Could you check a few things on this model? Use its own coordinates, in mm. A direction names the side the tool comes from. Give positions to 0.01 mm unless a question says otherwise; leave off trailing zeros. Order: outer loops, then holes, each group sorted by start corner. A loop starts at its lowest first (then second) coordinate and runs counter-clockwise, first axis right, second up. Notation, with made-up numbers: (-26, -0.5) - (32, -0.5) arc R16 cw to (32, 16.5) - close; hole circle Ø7 at (2.5, 88.5). An arc over 180 degrees is marked (long way). One line per question, with ' | ' between items. Start each with the question number.
1. I need wall thicknesses on probe 1 along Y at (x, z) = (-33.79, 13.25); probe 2 along X at (y, z) = (-1.5, 16.25) (3 decimals); probe 3 along Y at (x, z) = (-26.5, 4.75). Which ranges of each line are inside material? Lowest first, please. Write a range as from..to.
2. Imagine slicing it at C-C (z = 16). Please give me the cut outline in (x, y) (3 decimals).
3. Imagine slicing it at D-D (z = 8.75). Please give me the cut outline in (x, y) (3 decimals), and give its area (3 significant figures).
4. Which directions (+Z, -Z, +X, -X, +Y, -Y) give clear straight access to the entire face, cutting with the end or side of a thin tool? Please do faces 4 (the flat face through (-10, 10.4, 10)), 5 (the cylindrical face through (12.65, 4.19, 14.85)), 6 (the flat face through (22.395, 3, 10)).
5. Imagine slicing it at A-A (y = -4.9). Please give me the cut outline in (x, z) (3 decimals), and give its area (3 significant figures).
6. Imagine slicing it at B-B (x = 14.89). Please give me the cut outline in (y, z), and give its area (3 significant figures).
7. If we mould it in two halves opening along X, with no side actions, what happens to faces 1 (the flat face through (-41.395, 3, 10)), 2 (the flat face through (15, -5, 10)), 3 (the flat face through (-10, 11, 20))? For each: released by +X, released by -X, zero draft, split by the parting line, or undercut.
8. For P1, Ø10, axis at x = -0.5, y = 8.5, coming from the +Z side; P2, Ø5, axis at x = 14.5, y = -5, coming from the +Z side; P3, Ø3, axis at x = 14.89, y = -4.9, coming from the +Z side; P4, Ø6, axis at x = -33.79, y = -4.9, coming from the +Z side, each with a flat end and sliding along its axis, tell me the tip position at first contact or that it passes through.
```python
from build123d import *

# Parameters (mm, degrees)
SKETCH1_W           = 18.495
SKETCH1_H           = 20.8
SKETCH1_W_2         = 10
SKETCH1_W_3         = 37.395
BOSS_EXTRUDE1_DEPTH = 20
SKETCH6_W           = 106.79
SKETCH6_H           = 20
BOSS_EXTRUDE4_DEPTH = 5
SKETCH9_R           = 2.35
CUT_EXTRUDE1_DEPTH  = 10
SKETCH10_W          = 20
SKETCH10_H          = 25.8
CUT_EXTRUDE2_DEPTH  = 17
SKETCH11_W          = 20
SKETCH11_H          = 25.8
CUT_EXTRUDE3_DEPTH  = 26
CHAMFER1_SIZE       = 1
CHAMFER1_SIZE2      = 0.424474816


with BuildPart() as part:
    # Sketch1 → Boss-Extrude1 (new body)
    with BuildSketch(Plane.XY):
        with Locations((-39.1475, 0)):
            Rectangle(SKETCH1_W, SKETCH1_H)
        with Locations((-53.395, 0)):
            Rectangle(SKETCH1_W_2, SKETCH1_H)
        with Locations((29.6975, 0)):
            Rectangle(SKETCH1_W_3, SKETCH1_H)
    extrude(amount=BOSS_EXTRUDE1_DEPTH)

    # Sketch6 → Boss-Extrude4 (add)
    with BuildSketch(Plane(origin=(0, 10.4, 0), x_dir=(1, 0, 0), z_dir=(0, 1, 0))):
        with Locations((-5, -10)):
            Rectangle(SKETCH6_W, SKETCH6_H)
    extrude(amount=BOSS_EXTRUDE4_DEPTH)

    # Sketch9 → Cut-Extrude1 (cut)
    with BuildSketch(Plane.XY.offset(20)):
        with Locations((14.89, -4.9)):
            Circle(SKETCH9_R)
        with Locations(Location((14.89, 4.9, 0), (0, 0, 180))):
            Circle(SKETCH9_R)
        with Locations(Location((-33.79, -4.9, 0), (0, 0, 180))):
            Circle(SKETCH9_R)
        with Locations((-33.79, 4.9)):
            Circle(SKETCH9_R)
    extrude(amount=-CUT_EXTRUDE1_DEPTH, mode=Mode.SUBTRACT)

    # Sketch10 → Cut-Extrude2 (cut)
    with BuildSketch(Plane.ZY.offset(58.395)):
        with Locations((10, 2.5)):
            Rectangle(SKETCH10_W, SKETCH10_H)
    extrude(amount=-CUT_EXTRUDE2_DEPTH, mode=Mode.SUBTRACT)

    # Sketch11 → Cut-Extrude3 (cut)
    with BuildSketch(Plane(origin=(48.395, 0, 0), x_dir=(0, 0, -1), z_dir=(1, 0, 0))):
        with Locations((-10, 2.5)):
            Rectangle(SKETCH11_W, SKETCH11_H)
    extrude(amount=-CUT_EXTRUDE3_DEPTH, mode=Mode.SUBTRACT)

    # Chamfer1
    chamfer1_edges = [part.edges().sort_by_distance(p)[0] for p in [
        (17.24, 4.9, 20),
        (-31.44, -4.9, 20),
        (-36.14, 4.9, 20),
        (12.54, -4.9, 20),
    ]]
    chamfer1_side = [part.faces().sort_by_distance(p)[0] for p in [
        (-35.6475, -9.711900872, 20),
    ]]
    chamfer(chamfer1_edges, length=CHAMFER1_SIZE, length2=CHAMFER1_SIZE2, reference=chamfer1_side[0])


solid = part.part
```
Results found:
1) probe 1: y = -10.4..-7.25, -2.55..2.55, 7.25..15.4 | probe 2: x = -41.395..-29.9, 11..22.395 | probe 3: y = 10.4..15.4
2) outline: (-41.395, -10.4) - (-29.9, -10.4) - (-29.9, 10.4) - (11, 10.4) - (11, -10.4) - (22.395, -10.4) - (22.395, 15.4) - (-41.395, 15.4) - close; hole circle Ø4.7 at (-33.79, -4.9); hole circle Ø4.7 at (-33.79, 4.9); hole circle Ø4.7 at (14.89, -4.9); hole circle Ø4.7 at (14.89, 4.9)
3) outline: (-41.395, -10.4) - (-29.9, -10.4) - (-29.9, 10.4) - (11, 10.4) - (11, -10.4) - (22.395, -10.4) - (22.395, 15.4) - (-41.395, 15.4) - close | area: 795 mm2
4) face 4: +Z, -Z, -Y | face 5: +Z | face 6: +Z, -Z, +X, +Y, -Y
5) outline: (-41.395, 0) - (-29.9, 0) - (-29.9, 20) - (-30.44, 20) - (-31.44, 19.576) - (-31.44, 10) - (-36.14, 10) - (-36.14, 19.576) - (-37.14, 20) - (-41.395, 20) - close; (11, 0) - (22.395, 0) - (22.395, 20) - (18.24, 20) - (17.24, 19.576) - (17.24, 10) - (12.54, 10) - (12.54, 19.576) - (11.54, 20) - (11, 20) - close | area: 363 mm2
6) outline: (-10.4, 0) - (15.4, 0) - (15.4, 20) - (8.25, 20) - (7.25, 19.58) - (7.25, 10) - (2.55, 10) - (2.55, 19.58) - (1.55, 20) - (-1.55, 20) - (-2.55, 19.58) - (-2.55, 10) - (-7.25, 10) - (-7.25, 19.58) - (-8.25, 20) - (-10.4, 20) - close | area: 421 mm2
7) face 1: released by -X | face 2: undercut | face 3: zero draft
8) P1: stops at z = 20 | P2: stops at z = 19.81 | P3: stops at z = 10 | P4: stops at z = 19.85
